from build123d import *

# Parameters (mm, degrees)
SKETCH1_R           = 9.525
BOSS_EXTRUDE1_DEPTH = 12.7
SKETCH2_W           = 5.08
SKETCH2_H           = 5.08
CUT_EXTRUDE2_DEPTH  = 6.35
BOSS_EXTRUDE2_DEPTH = 6.35
FILLET2_R           = 6.35
CUT_EXTRUDE3_REACH  = 14.065
SKETCH5_R           = 1.5875
SKETCH4_R           = 3.175
BOSS_EXTRUDE3_DEPTH = 6.35
DOME1_FACE_RADIUS   = 3.175
DOME1_HEIGHT        = 10.16


with BuildPart() as part:
    # Sketch1 → Boss-Extrude1 (new body)
    with BuildSketch(Plane.XY):
        Circle(SKETCH1_R)
    extrude(amount=BOSS_EXTRUDE1_DEPTH)

    # Sketch2 → Cut-Extrude2 (cut)
    with BuildSketch(Plane.XY.offset(12.7)):
        Rectangle(SKETCH2_W, SKETCH2_H)
    extrude(amount=-CUT_EXTRUDE2_DEPTH, mode=Mode.SUBTRACT)

    # Sketch3 → Boss-Extrude2 (add)
    with BuildSketch(Plane(origin=(0, 0, 0), x_dir=(-1, 0, 0), z_dir=(0, 0, -1))):
        with BuildLine():
            Line((-6.35, 10.172076103), (-6.35, 7.099515829))
            Line((-6.35, 7.099515829), (6.35, 7.099515829))
            Line((6.35, 7.099515829), (6.35, 10.172076103))
            Line((6.35, 10.172076103), (6.35, 86.372076103))
            ThreePointArc((6.35, 86.372076103), (0, 92.722076103), (-6.35, 86.372076103))
            Line((-6.35, 86.372076103), (-6.35, 10.172076103))
        make_face()
    extrude(amount=-BOSS_EXTRUDE2_DEPTH)

    # Fillet2
    fillet2_edges = [part.edges().sort_by_distance(p)[0] for p in [
        (-6.35, 7.099515829, 3.175),
        (6.35, 7.099515829, 3.175),
    ]]
    fillet(fillet2_edges, radius=FILLET2_R)

    # Sketch5 → Cut-Extrude3 (cut, up to next)
    with BuildSketch(Plane.ZY.offset(-2.54), mode=Mode.PRIVATE) as cut_extrude3_sk1:
        with Locations((9.525, 0)):
            Circle(SKETCH5_R)
    cut_extrude3_tool1 = extrude(cut_extrude3_sk1.sketch, amount=CUT_EXTRUDE3_REACH, mode=Mode.PRIVATE) & part.part
    add(cut_extrude3_tool1.solids().sort_by_distance((2.54, 0, 9.525))[0], mode=Mode.SUBTRACT)

    # Sketch4 → Boss-Extrude3 (add)
    with BuildSketch(Plane(origin=(0, 0, 0), x_dir=(-1, 0, 0), z_dir=(0, 0, -1))):
        with Locations((0, 86.372076103)):
            Circle(SKETCH4_R)
    extrude(amount=BOSS_EXTRUDE3_DEPTH)

    # Dome1: a dome of height H over a round flat face of radius A is a cap of a sphere of radius (A * A + H * H) / (2 * H)
    dome1_r = (DOME1_FACE_RADIUS * DOME1_FACE_RADIUS + DOME1_HEIGHT * DOME1_HEIGHT) / (2 * DOME1_HEIGHT)
    dome1_base = Plane((0, 86.372076103, -6.35), z_dir=(0, 0, -1))
    with Locations(dome1_base.offset(DOME1_HEIGHT - dome1_r)):
        dome1_ball = Sphere(dome1_r, mode=Mode.PRIVATE)
    add(split(dome1_ball, bisect_by=dome1_base, keep=Keep.TOP, mode=Mode.PRIVATE))


solid = part.part
Verification items for the finished model (mm, model axes). A direction names the side the tool comes from. Coordinates: 2 decimals unless noted, no trailing zeros. Order: outer loops, then holes, each group sorted by start corner. A loop starts at its lowest first (then second) coordinate and runs counter-clockwise, first axis right, second up. Notation, with made-up numbers: M 66.5,66.25 L 109.5,66.25 A14 cw 109.5,93.25 Z; hole C -24,-15 d8. An arc over 180 degrees is marked long. Write each question's results on one line, items separated by ' | '.
1) Scan lines: line 1 along Z through (x, y) = (-6, 0); line 2 along Z through (x, y) = (3.25, 34); line 3 along X through (y, z) = (27, 5.75). Record each from-to range of solid material in increasing order. Write a range as [from, to].
Solved:
line 1: z = [0, 7.94], [11.11, 12.7] | line 2: z = [0, 6.35] | line 3: x = [-6.35, 6.35]
2) Gauge pin test, flat ends, axial feed: pin 1 Ø1.5 at (x, z) = (2, -10) entering from -Y; pin 2 Ø1.5 at (y, z) = (1, 10) entering from -X; pin 3 Ø1 at (y, z) = (1, 5.5) entering from +X. Record the tip position at first contact, or that the pin passes through.
Solved:
pin 1: stops at y = 80.99 | pin 2: stops at x = -9.47 | pin 3: stops at x = 9.51
3) Section check C-C on x = 4.5. Record the cut outline in (y, z).
Solved:
outline: M -8.39,0 L 90.85,0 L 90.85,6.35 L 8.39,6.35 L 8.39,12.7 L -8.39,12.7 Z; C 86.37,-10.93 d6.59
4) Section check D-D on z = -4.75. Record the cut outline in (x, y) (3 decimals), plus the area to 3 significant figures.
Solved:
outline: C 0,86.372 d6.35 | area: 31.7 mm²
5) Section check B-B on x = 0. Record the cut outline in (y, z) (3 decimals), plus the area to 3 significant figures.
Solved:
outline: M -9.525,0 L 83.197,0 L 83.197,-6.35 A5.576 ccw long 89.547,-6.35 L 89.547,0 L 92.722,0 L 92.722,6.35 L 9.525,6.35 L 9.525,12.7 L 2.54,12.7 L 2.54,6.35 L -2.54,6.35 L -2.54,12.7 L -9.525,12.7 Z | area: 872 mm²
6) Access from +Z, -Z, +X, -X, +Y, -Y to the whole of each face (thin tool, end or side, straight path). Record for faces 1 (the face through (4.4, -8.45, 6.26)), 2 (the face through (-5.98, 0.07, 7.94)), 3 (the face through (6.35, 48, 3)), 4 (the face through (-1.707, 89.049, -3.131)).
Solved:
face 1: +Z | face 2: -X | face 3: +Z, -Z, +X, +Y | face 4: none
7) Release check for a two-part mould opening along X. For faces 5 (the face through (-6.35, 47, 3)), 6 (the face through (0, 31, 0)), 7 (the face through (-2.54, -2, 10)) record: pulls with the +X half, pulls with the -X half, needs draft (parallel to the pull), parting line crosses it, or undercut.
Solved:
face 5: pulls with the -X half | face 6: needs draft | face 7: undercut
